The listing builds one solid part. Answer for the finished solid, in the listing's coordinates (mm). Give positions to 0.01 mm unless a question says otherwise; leave off trailing zeros. Loops run counter-clockwise (first coordinate to the right, second up) from the corner with the lowest first, then second, coordinate; pieces in that order, holes last. Notation, with made-up numbers: (-24, 34.5) - (-12, 34.5) arc R19 ccw to (-12, 49.5) - close; hole circle Ø10 at (-40, -11). An arc over 180 degrees is marked (long way). Write each question's results on one line, items separated by ' | '.
from build123d import *

# Parameters (mm, degrees)
SKETCH1_W           = 30
SKETCH1_H           = 36.83
SKETCH1_R           = 2.1
BOSS_EXTRUDE1_DEPTH = 4
CHAMFER1_SIZE       = 7.5
SKETCH2_R           = 1.6
CUT_EXTRUDE1_DEPTH  = 48.670209775


with BuildPart() as part:
    # Sketch1 → Boss-Extrude1 (new body)
    with BuildSketch(Plane(origin=(0, 0, 0), x_dir=(1, 0, 0), z_dir=(0, 1, 0))):
        with Locations((15, 18.415)):
            Rectangle(SKETCH1_W, SKETCH1_H)
        with Locations(Location((5, 23.415, 0), (0, 0, 270))):
            Circle(SKETCH1_R, mode=Mode.SUBTRACT)
        with Locations(Location((5, 13.415, 0), (0, 0, 270))):
            Circle(SKETCH1_R, mode=Mode.SUBTRACT)
    extrude(amount=BOSS_EXTRUDE1_DEPTH)

    # Chamfer1
    chamfer1_edges = [part.edges().sort_by_distance(p)[0] for p in [
        (0, 2, -36.83),
        (0, 2, 0),
    ]]
    chamfer(chamfer1_edges, length=CHAMFER1_SIZE)

    # Sketch2 → Cut-Extrude1 (cut, through all)
    with BuildSketch(Plane(origin=(0, 4, 0), x_dir=(1, 0, 0), z_dir=(0, 1, 0))):
        with Locations(Location((20, 29.377825135, 0), (0, 0, 270))):
            Circle(SKETCH2_R)
        with Locations(Location((20, 7.716339326, 0), (0, 0, 270))):
            Circle(SKETCH2_R)
    extrude(amount=-CUT_EXTRUDE1_DEPTH, mode=Mode.SUBTRACT)


solid = part.part
Item 1: Find the intervals of material crossed by line 1 along Z through (x, y) = (5.5, 0.25); line 2 along X through (y, z) = (1.9, -23.5); line 3 along X through (y, z) = (2.75, -28.5), in increasing order. Write a range as [from, to].
Values found:
line 1: z = [-34.83, -25.45], [-21.38, -15.45], [-11.38, -2] | line 2: x = [0, 2.9], [7.1, 30] | line 3: x = [0, 18.66], [21.34, 30]
Item 2: A flat-ended cylindrical pin translates along its axis: P1, Ø2.5, axis at x = 5, z = -13.415, coming from the +Y side. Find the tip coordinate at first contact, or state that the pin passes through.
Values found:
P1: passes through
Item 3: A cutting plane is placed at A-A, the plane x = 20. Determine the outline of the cut face in (y, z), plus the area to 3 significant figures.
Values found:
outline: (0, -36.83) - (4, -36.83) - (4, -30.98) - (0, -30.98) - close; (0, -27.78) - (4, -27.78) - (4, -9.32) - (0, -9.32) - close; (0, -6.12) - (4, -6.12) - (4, 0) - (0, 0) - close | area: 122 mm²
Item 4: A cutting plane is placed at B-B, the plane z = -24. Determine the outline of the cut face in (x, y).
Values found:
outline: (0, 0) - (2.98, 0) - (2.98, 4) - (0, 4) - close; (7.02, 0) - (30, 0) - (30, 4) - (7.02, 4) - close
Item 5: For a pull along Z with two mould halves and no side action, classify faces 1 (the face through (30, 2, -18)), 2 (the face through (3.8, 1.97, -33.13)), 3 (the face through (5.63, 1.97, -21.41)), 4 (the face through (3.8, 2, -3.7)) as released by +Z, released by -Z, zero draft, split by the parting line, or undercut.
Values found:
face 1: zero draft | face 2: released by -Z | face 3: undercut | face 4: released by +Z
Item 6: A cutting plane is placed at D-D, the plane x = 5. Determine the outline of the cut face in (y, z) (3 decimals).
Values found:
outline: (0, -34.33) - (4, -34.33) - (4, -25.515) - (0, -25.515) - close; (0, -21.315) - (4, -21.315) - (4, -15.515) - (0, -15.515) - close; (0, -11.315) - (4, -11.315) - (4, -2.5) - (0, -2.5) - close
Item 7: A cutting plane is placed at C-C, the plane y = 0.75. Determine the outline of the cut face in (x, z) (3 decimals), plus the area to 3 significant figures.
Values found:
outline: (0, -29.33) - (7.5, -36.83) - (30, -36.83) - (30, 0) - (7.5, 0) - (0, -7.5) - close; hole circle Ø4.2 at (5, -23.415); hole circle Ø4.2 at (5, -13.415); hole circle Ø3.2 at (20, -29.378); hole circle Ø3.2 at (20, -7.716) | area: 1,000 mm²
